Design review of the part built by this model. Coordinates are the model's own, in mm. A direction names the side the tool comes from. Coordinates: 2 decimals unless noted, no trailing zeros. Order: outer loops, then holes, each group sorted by start corner. A loop starts at its lowest first (then second) coordinate and runs counter-clockwise, first axis right, second up. Notation, with made-up numbers: (9.25, -38) -> (52.25, -38) arc R25 ccw to (52.25, -8) -> close; hole circle Ø10 at (12.25, 10.5). An arc over 180 degrees is marked (long way). Use a Markdown table: item, result. Add a question column.
Q1. Machinability: for faces 4 (the face through (-3, 0, -54)), 5 (the face through (-3, 0.914, -54)), which of the approach directions +Z, -Z, +X, -X, +Y, -Y give a long, thin tool a straight path to every point of the face, cutting with its end or side? Answer none if there is none.
Q2. Insertion check: pin 1 (10 mm diameter, centred on x = -34, y = 3.5, fed in from +Z); pin 2 (6 mm diameter, centred on y = 13.61, z = 88.9, fed in from -X); pin 3 (2 mm diameter, centred on x = -101.5, z = -75, fed in from +Y). Each pin has a flat end and moves straight along its axis. Give the tip position at first contact, or say it passes through.
Q3. Add section A-A (z = 46). State the section outline as (x, y) points, then the cut area to 3 significant figures.
Q4. Add section B-B (x = -160.5). State the section outline as (y, z) points, then the cut area to 3 significant figures.
Q5. The part is to be moulded in two halves that separate along X. For faces 1 (the face through (233.629, 11, 3)), 2 (the face through (-233.629, 11, -3)), 3 (the face through (-232.715, 16, -3)), say which applies: pulls with the +X half, pulls with the -X half, needs draft (parallel to the pull), parting line crosses it, or undercut.
Q6. Wall thickness on probe 1 along X at (y, z) = (7.5, 16.5); probe 2 along Y at (x, z) = (-43.5, 127); probe 3 along Y at (x, z) = (233, -88): over which ranges is each line inside the solid? List them lowest first.
from build123d import *

# Parameters (mm, degrees)
SKETCH1_W                    = 465.4296
SKETCH1_H                    = 457.2
BOSS_EXTRUDE1_DEPTH          = 0.9144
EDGE_FLANGE1_STRIP_W         = 5.4864
EDGE_FLANGE1_STRIP_H         = 0.9144
EDGE_FLANGE1_STRIP_CUT_DEPTH = 457.2
EDGE_FLANGE1_DEPTH           = 457.2
EDGE_FLANGE2_STRIP_W         = 5.4864
EDGE_FLANGE2_STRIP_H         = 0.9144
EDGE_FLANGE2_STRIP_CUT_DEPTH = 457.2
EDGE_FLANGE2_DEPTH           = 457.2
CUT_EXTRUDE1_START           = -233.6292
CUT_EXTRUDE1_OUTLINE_R       = 3.2639
CUT_EXTRUDE1_DEPTH           = 467.2584
CUT_EXTRUDE1_START_2         = -0.9144
CUT_EXTRUDE1_2_OUTLINE_R     = 21.082
CUT_EXTRUDE1_2_DEPTH         = 0.9144


# Read off the part's stored shape, not the designer's step: Cut-Extrude1
# Sheet-metal steps are written as plain solids
with BuildPart() as part:
    # Sketch1 → Boss-Extrude1 (new body)
    with BuildSketch(Plane(origin=(0, 0, 0), x_dir=(1, 0, 0), z_dir=(0, 1, 0))):
        Rectangle(SKETCH1_W, SKETCH1_H)
    extrude(amount=BOSS_EXTRUDE1_DEPTH)

    # Edge-Flange1 strip (across the edge) → Edge-Flange1 strip cut (cut)
    with BuildSketch(Plane(origin=(-232.7148, 0.9144, -228.6), x_dir=(1, 0, 0), z_dir=(0, 0, 1))):
        with Locations((-1.8288, -0.4572)):
            Rectangle(EDGE_FLANGE1_STRIP_W, EDGE_FLANGE1_STRIP_H)
    extrude(amount=EDGE_FLANGE1_STRIP_CUT_DEPTH, mode=Mode.SUBTRACT)

    # Edge-Flange1 section (across the edge) → Edge-Flange1 (add)
    with BuildSketch(Plane(origin=(-232.7148, 0.9144, -228.6), x_dir=(1, 0, 0), z_dir=(0, 0, 1))):
        with BuildLine():
            Line((-0.9144, 0.9144), (-0.9144, 24.4856))
            Line((-0.9144, 24.4856), (0, 24.4856))
            Line((0, 24.4856), (0, 0.9144))
            ThreePointArc((0, 0.9144), (0.267821559, 0.267821559), (0.9144, 0))
            Line((0.9144, 0), (0.9144, -0.9144))
            ThreePointArc((0.9144, -0.9144), (-0.378756881, -0.378756881), (-0.9144, 0.9144))
        make_face()
    extrude(amount=EDGE_FLANGE1_DEPTH)

    # Edge-Flange2 strip (across the edge) → Edge-Flange2 strip cut (cut)
    with BuildSketch(Plane(origin=(232.7148, 0.9144, 228.6), x_dir=(-1, 0, 0), z_dir=(0, 0, -1))):
        with Locations((-1.8288, -0.4572)):
            Rectangle(EDGE_FLANGE2_STRIP_W, EDGE_FLANGE2_STRIP_H)
    extrude(amount=EDGE_FLANGE2_STRIP_CUT_DEPTH, mode=Mode.SUBTRACT)

    # Edge-Flange2 section (across the edge) → Edge-Flange2 (add)
    with BuildSketch(Plane(origin=(232.7148, 0.9144, 228.6), x_dir=(-1, 0, 0), z_dir=(0, 0, -1))):
        with BuildLine():
            Line((-0.9144, 0.9144), (-0.9144, 24.4856))
            Line((-0.9144, 24.4856), (0, 24.4856))
            Line((0, 24.4856), (0, 0.9144))
            ThreePointArc((0, 0.9144), (0.267821559, 0.267821559), (0.9144, 0))
            Line((0.9144, 0), (0.9144, -0.9144))
            ThreePointArc((0.9144, -0.9144), (-0.378756881, -0.378756881), (-0.9144, 0.9144))
        make_face()
    extrude(amount=EDGE_FLANGE2_DEPTH)

    # Cut-Extrude1 outline → Cut-Extrude1 (cut)
    with BuildSketch(Plane.YZ.offset(CUT_EXTRUDE1_START)):
        with Locations((13.6144, -177.8)):
            Circle(CUT_EXTRUDE1_OUTLINE_R)
        with Locations((13.6144, -88.9)):
            Circle(CUT_EXTRUDE1_OUTLINE_R)
        with Locations((13.6144, 0)):
            Circle(CUT_EXTRUDE1_OUTLINE_R)
        with Locations((13.6144, 88.9)):
            Circle(CUT_EXTRUDE1_OUTLINE_R)
        with Locations((13.6144, 177.8)):
            Circle(CUT_EXTRUDE1_OUTLINE_R)
    extrude(amount=CUT_EXTRUDE1_DEPTH, mode=Mode.SUBTRACT)

    # Cut-Extrude1 2 outline → Cut-Extrude1 2 (cut)
    with BuildSketch(Plane(origin=(0, 0.9144, 0), x_dir=(1, 0, 0), z_dir=(0, 1, 0)).offset(CUT_EXTRUDE1_START_2)):
        with Locations((-0.39878, -11.1252)):
            Circle(CUT_EXTRUDE1_2_OUTLINE_R)
    extrude(amount=CUT_EXTRUDE1_2_DEPTH, mode=Mode.SUBTRACT)


solid = part.part
Established:
| question | item | result |
|---|---|---|
| 1 | face 4 | +Z, -Z, +X, -X, -Y |
| 1 | face 5 | +Z, -Z, +Y |
| 2 | pin 1 | z = 228.6 |
| 2 | pin 2 | through |
| 2 | pin 3 | y = 0.91 |
| 3 | outline | (-233.63, 1.83) arc R1.83 ccw to (-231.8, 0) -> (231.8, 0) arc R1.83 ccw to (233.63, 1.83) -> (233.63, 25.4) -> (232.71, 25.4) -> (232.71, 1.83) arc R0.91 cw to (231.8, 0.91) -> (-231.8, 0.91) arc R0.91 cw to (-232.71, 1.83) -> (-232.71, 25.4) -> (-233.63, 25.4) -> close |
| 3 | area | 471 mm^2 |
| 4 | outline | (0, -228.6) -> (0.91, -228.6) -> (0.91, 228.6) -> (0, 228.6) -> close |
| 4 | area | 418 mm^2 |
| 5 | face 1 | pulls with the +X half |
| 5 | face 2 | pulls with the -X half |
| 5 | face 3 | undercut |
| 6 | probe 1 | -233.63 to -232.71, 232.71 to 233.63 |
| 6 | probe 2 | 0 to 0.91 |
| 6 | probe 3 | 0.45 to 10.48, 16.75 to 25.4 |
